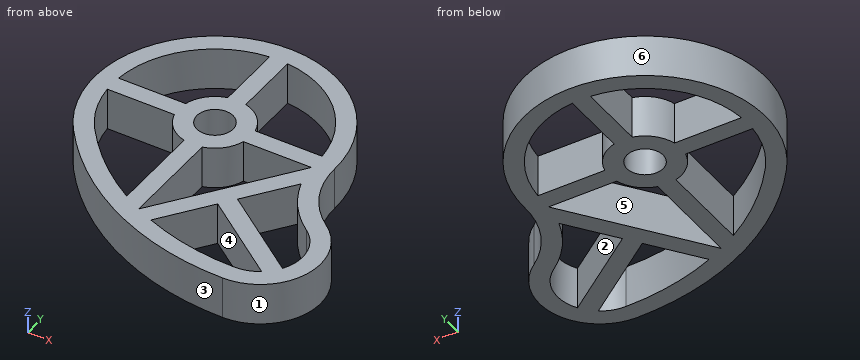
from build123d import *

# Parameters (mm, degrees)
SKETCH1_R           = 3
BOSS_EXTRUDE2_DEPTH = 7
CUT_EXTRUDE2_DEPTH  = 10


with BuildPart() as part:
    # Sketch1 → Boss-Extrude2 (new body)
    with BuildSketch(Plane.XY):
        with BuildLine():
            ThreePointArc((19.998941051, -0.20580779), (-6.226847104, 19.005956307), (-16, -12))
            ThreePointArc((-16, -12), (-0.124611797, -25.249223595), (20, -30))
            ThreePointArc((20, -30), (29.509457722, -23.09357622), (25.883646455, -11.914042766))
            ThreePointArc((25.883646455, -11.914042766), (21.521016167, -6.773774564), (19.998941051, -0.20580779))
        make_face()
        Circle(SKETCH1_R, mode=Mode.SUBTRACT)
    extrude(amount=BOSS_EXTRUDE2_DEPTH)

    # Sketch4 → Cut-Extrude2 (cut)
    with BuildSketch(Plane.XY):
        with BuildLine():
            Line((-1.5, -21.079772727), (-1.5, -5.809475019))
            ThreePointArc((-1.5, -5.809475019), (-4.242640687, -4.242640687), (-5.809475019, -1.5))
            Line((-5.809475019, -1.5), (-16.933694222, -1.5))
            ThreePointArc((-16.933694222, -1.5), (-15.874480171, -6.082834807), (-13.6, -10.2))
            ThreePointArc((-13.6, -10.2), (-8.081931266, -16.231476692), (-1.5, -21.079772727))
        make_face()
        with BuildLine():
            ThreePointArc((-5.809475019, 1.5), (-4.242640687, 4.242640687), (-1.5, 5.809475019))
            Line((-1.5, 5.809475019), (-1.5, 16.933694222))
            ThreePointArc((-1.5, 16.933694222), (-12.02081528, 12.02081528), (-16.933694222, 1.5))
            Line((-16.933694222, 1.5), (-5.809475019, 1.5))
        make_face()
        with BuildLine():
            ThreePointArc((1.5, 5.809475019), (4.305801895, 4.178524864), (5.851855009, 1.325063379))
            Line((5.851855009, 1.325063379), (16.948280356, 1.325063379))
            ThreePointArc((16.948280356, 1.325063379), (12.082719116, 11.958591003), (1.5, 16.933694222))
            Line((1.5, 16.933694222), (1.5, 5.809475019))
        make_face()
        with BuildLine():
            Line((17.048775601, -1.674936621), (5.761474405, -1.674936621))
            ThreePointArc((5.761474405, -1.674936621), (4.178020413, -4.306291377), (1.5, -5.809475019))
            Line((1.5, -5.809475019), (1.5, -22.706100302))
            Line((1.5, -22.706100302), (17.048775601, -1.674936621))
        make_face()
        with BuildLine():
            ThreePointArc((24.118552518, -14.339829936), (20.286608679, -10.499414856), (17.832718736, -5.660922764))
            Line((17.832718736, -5.660922764), (12.106553004, -13.40609395))
            Line((12.106553004, -13.40609395), (25.969739669, -23.655435444))
            ThreePointArc((25.969739669, -23.655435444), (26.865750965, -18.635645321), (24.118552518, -14.339829936))
        make_face()
        with BuildLine():
            Line((10.323082943, -15.818402915), (4.305668643, -23.95751485))
            ThreePointArc((4.305668643, -23.95751485), (12.00674108, -26.232363646), (20, -27))
            ThreePointArc((20, -27), (22.020668793, -26.702006985), (23.869296105, -25.833399322))
            Line((23.869296105, -25.833399322), (10.323082943, -15.818402915))
        make_face()
    extrude(amount=CUT_EXTRUDE2_DEPTH, mode=Mode.SUBTRACT)


solid = part.part
Here's how the part is built. I have some questions about the finished solid (model axes, mm). Face numbers are marked on the shaded views. A direction names the side the tool comes from. Give positions to 0.01 mm unless a question says otherwise; leave off trailing zeros. Loops run counter-clockwise (first coordinate to the right, second up) from the corner with the lowest first, then second, coordinate; pieces in that order, holes last. Notation, with made-up numbers: (89, -28) -> (136, -28) arc R33 ccw to (136, 0) -> close; hole circle Ø6 at (78, 8.25). An arc over 180 degrees is marked (long way). One line per item, written item: value.
Q1. Suppose I cut it at D-D on x = 0. Please give me the cut outline in (y, z).
Answers follow:
outline: (-25.31, 0) -> (-3, 0) -> (-3, 7) -> (-25.31, 7) -> close; (3, 0) -> (20, 0) -> (20, 7) -> (3, 7) -> close
Q2. I'm going to push flat-ended pins straight in: pin 1 Ø2 at (y, z) = (-15, 2) entering from -X; pin 2 Ø3.5 at (y, z) = (9, 3) entering from +X; pin 3 Ø3.5 at (x, z) = (9.5, 4) entering from +Y. Where does each tip first touch, or does it pass through?
Answers follow:
pin 1: x = -14.41
pin 2: x = 18.64
pin 3: y = 18.44
Q3. We'd pull the mould along Y, two halves only. Please class the marked faces 3, 4, 5 and 6: pulls with the +Y half, pulls with the -Y half, needs draft (parallel to the pull), parting line crosses it, or undercut.
Answers follow:
face 3: pulls with the -Y half
face 4: undercut
face 5: undercut
face 6: parting line crosses it
Q4. Suppose I cut it at C-C on z = 6.25. State how many separate pieces and enclosed holes the cut face has, then the cut area to 3 significant figures.
Answers follow:
separate pieces: 1
enclosed holes: 7
area: 798 mm^2
Q5. Suppose I cut it at A-A on y = 8. Please give me the cut outline in (x, z).
Answers follow:
outline: (-18.33, 0) -> (-15, 0) -> (-15, 7) -> (-18.33, 7) -> close; (-1.5, 0) -> (1.5, 0) -> (1.5, 7) -> (-1.5, 7) -> close; (15, 0) -> (18.33, 0) -> (18.33, 7) -> (15, 7) -> close
Q6. If I drill on line 1 along X through (y, z) = (-19, 2); line 2 along X through (y, z) = (9.5, 2); line 3 along Y through (x, z) = (10, 6.75), over which ranges is the centre line in solid material (lowest first)?
Answers follow:
line 1: -9.48 to -4.66, -1.5 to 1.5, 4.24 to 7.97, 14.63 to 19.67, 26.93 to 29.95
line 2: -17.6 to -14.1, -1.5 to 1.5, 14.1 to 17.6
line 3: -28.87 to -25.79, -16.26 to -11.21, -1.67 to 1.33, 13.75 to 17.32
Q7. On a 3-axis mill with a long thin cutter (end or side, diameter ignored), from which of +Z, -Z, +X, -X, +Y, -Y can I reach the whole of each face in a straight line? I mean the marked faces 1 and 2. Say none if no direction works.
Answers follow:
face 1: +Z, -Z, +X
face 2: +Z, -Z
Q8. Suppose I cut it at B-B on x = -7. Please give me the cut outline in (y, z) (3 decimals), then the cut area to 3 significant figures.
Answers follow:
outline: (-21, 0) -> (-17.171, 0) -> (-17.171, 7) -> (-21, 7) -> close; (-1.5, 0) -> (1.5, 0) -> (1.5, 7) -> (-1.5, 7) -> close; (15.492, 0) -> (18.735, 0) -> (18.735, 7) -> (15.492, 7) -> close
area: 70.5 mm^2
